Input: dimensioned drawing with shaded views. Units: mm. Origin: part minimum x, y, z. Coordinates: 2 decimals unless noted, no trailing zeros. Order: outer loops, then holes, each group sorted by start corner. A loop starts at its lowest first (then second) coordinate and runs counter-clockwise, first axis right, second up. Notation, with made-up numbers: M 63,-10.5 L 68,-10.5 A9 cw 68,4.5 Z; hole C -17.75,-32 d5. An arc over 180 degrees is marked long. Write item = value, one per line.
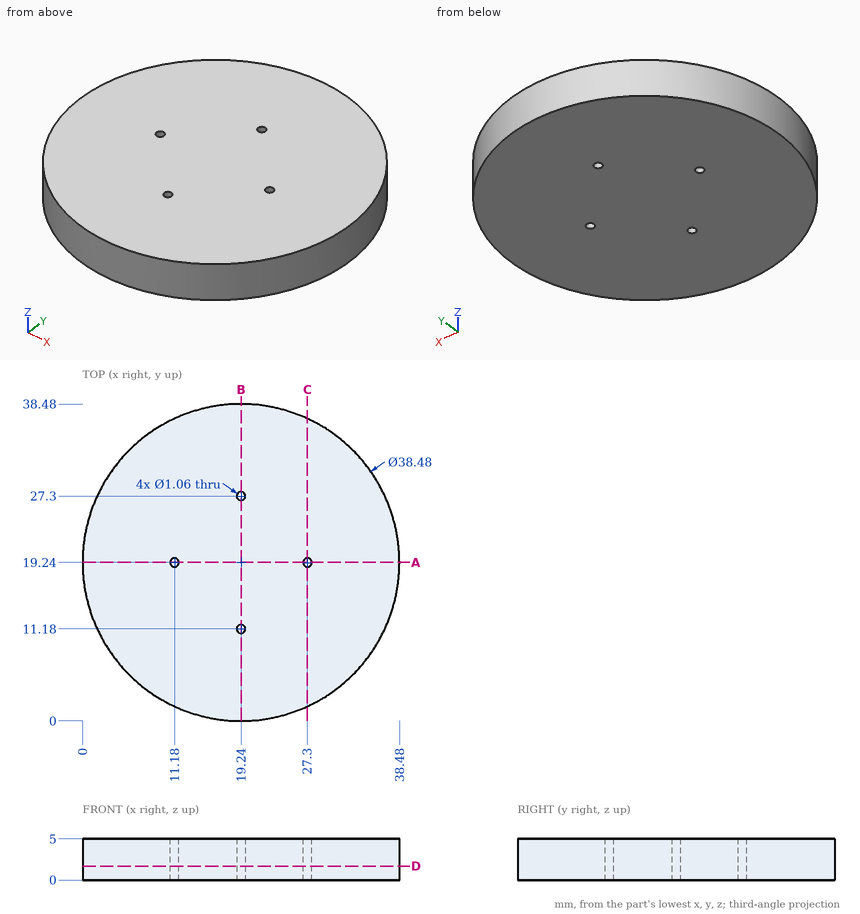
1) Pin query (flat end, axial travel): pin 1 (1.5 mm diameter, centred on x = 16.5, z = 2.5, fed in from +Y); pin 2 (1.5 mm diameter, centred on y = 22.5, z = 4, fed in from +X); pin 3 (1.5 mm diameter, centred on x = 8, z = 1, fed in from +Y). Return the tip coordinate at first contact, or that it passes through.
Numbers:
pin_1 = 38.38
pin_2 = 38.32
pin_3 = 35.37
2) Section A-A, the plane y = 19.24. Return loops of the section in (x, z), and give its area (3 significant figures).
Numbers:
outline = M 0,0 L 10.65,0 L 10.65,5 L 0,5 Z; M 11.71,0 L 26.77,0 L 26.77,5 L 11.71,5 Z; M 27.83,0 L 38.48,0 L 38.48,5 L 27.83,5 Z
area = 182 mm²
3) Section C-C, the plane x = 27.3. Return loops of the section in (y, z), and give its area (3 significant figures).
Numbers:
outline = M 1.77,0 L 18.71,0 L 18.71,5 L 1.77,5 Z; M 19.77,0 L 36.71,0 L 36.71,5 L 19.77,5 Z
area = 169 mm²
4) Section D-D, the plane z = 1.7. Return loops of the section in (x, y), and give its area (3 significant figures).
Numbers:
outline = C 19.24,19.24 d38.48; hole C 11.18,19.24 d1.06; hole C 19.24,11.18 d1.06; hole C 19.24,27.3 d1.06; hole C 27.3,19.24 d1.06
area = 1,160 mm²
5) Line query: L1, parallel to Y at x = 19.24, z = 3.6; L2, parallel to Y at x = 32, z = 2.2; L3, parallel to X at y = 5, z = 1.55. Output: solid intervals per line, ascending.
Numbers:
L1 = 0 to 10.65, 11.71 to 26.77, 27.83 to 38.48
L2 = 4.84 to 33.64
L3 = 6.3 to 32.18
